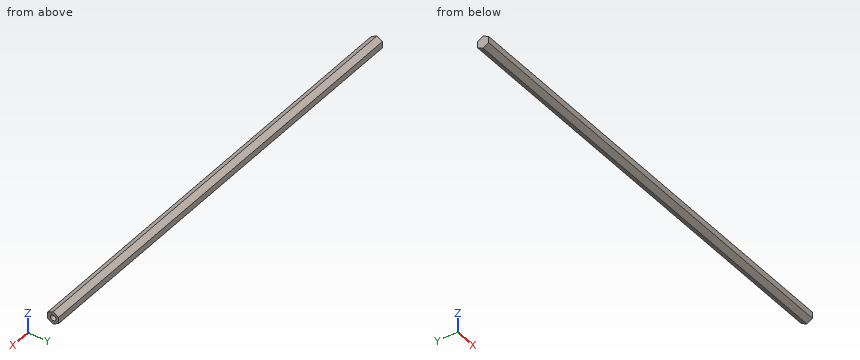
Autodesk Inventor part; units mm, degrees
ref_plane "YZ Plane" through (0, 0, 0) normal (1, 0, 0) x (0, 1, 0)
ref_plane "XZ Plane" through (0, 0, 0) normal (0, 1, 0) x (-1, 0, 0)
ref_plane "XY Plane" through (0, 0, 0) normal (0, 0, 1) x (1, 0, 0)
sketch "Sketch1" plane through (0, 0, 0) normal (1, 0, 0) x (0, 1, 0)
  line L0 (6.35, 3.6662) -> (6.35, -3.6662)
  line L1 (6.35, -3.6662) -> (0, -7.3323)
  line L2 (0, -7.3323) -> (-6.35, -3.6662)
  line L3 (-6.35, -3.6662) -> (-6.35, 3.6662)
  line L4 (-6.35, 3.6662) -> (0, 7.3323)
  line L5 (0, 7.3323) -> (6.35, 3.6662)
  point P0 (0, 0)
  dimension "d0" = 12.7
  dimension "d1" = 12.7
  dimension "d2" = 12.7
  dimension "d3" = 6.35
  dimension "d4" = 120
  dimension "d5" = 120
  dimension "d6" = 6.35
  dimension "d7" = 6.35
extrude "Extrusion1" add sketch "Sketch1" along normal blind 498.475
sketch "Sketch2" plane through (498.475, 0, 0) normal (1, 0, 0) x (0, 0, -1)
  circle A0 centre (0, 0) radius 3.175
  dimension "d10" = 6.35
extrude "Extrusion2" cut sketch "Sketch2" against normal blind 12.7
thread "Thread1"
properties part number "0.5 hex shaft" material "Steel, Alloy"
Geometry check sheet. Reference: the model listing, model coordinates, mm. Coordinates: 2 decimals unless noted, no trailing zeros. Write each loop counter-clockwise with the first axis right and the second up, starting at its lowest first coordinate (ties: lowest second). Pieces come first, ordered by that corner, then holes. Notation, with made-up numbers: (27, 12) -> (33, 12) arc R8 cw to (33, 17) -> close; hole circle Ø9 at (12.5, 16.5). An arc over 180 degrees is marked (long way). Use CSV: the item, a comma, the result in double quotes. Start each with the question number.
Item 1: Cross-section at A-A, the plane x = 461.5. Record the cut outline in (y, z), plus the area to 3 significant figures.
Item 2: Thickness scan on line 1 (Y direction, x = 495.5, z = 0) (3 decimals); line 2 (Z direction, x = 68, y = -1.75); line 3 (X direction, y = -2, z = -0.25) (3 decimals). Record the ranges inside material, lowest first.
Item 3: Depth check by flat-ended pin: pin 1 Ø4 at (x, y) = (224.5, 4) entering from +Z. Enter the tip coordinate at first touch or a pass-through.
Answers:
1,outline,"(-6.35, -3.67) -> (0, -7.33) -> (6.35, -3.67) -> (6.35, 3.67) -> (0, 7.33) -> (-6.35, 3.67) -> close"
1,area,"140 mm^2"
2,line 1,"-6.35 to -3.175, 3.175 to 6.35"
2,line 2,"-6.32 to 6.32"
2,line 3,"0 to 485.775"
3,pin 1,"z = 6.18"
